Autodesk Inventor part; units mm, degrees
ref_plane "YZ Plane" through (0, 0, 0) normal (1, 0, 0) x (0, 1, 0)
ref_plane "XZ Plane" through (0, 0, 0) normal (0, 1, 0) x (-1, 0, 0)
ref_plane "XY Plane" through (0, 0, 0) normal (0, 0, 1) x (1, 0, 0)
sketch "Sketch4" plane through (0, 0, 0) normal (0, 1, 0) x (-1, 0, 0)
  line L0 (0, -20.574) -> (0, -15.748)
  line L1 (0, -15.748) -> (-3.302, -15.748)
  line L2 (-3.302, -15.748) -> (-3.302, -16.764)
  line L3 (-3.302, -16.764) -> (-10.2362, -16.764)
  line L4 (-10.2362, -16.764) -> (-10.2362, -20.574)
  line L5 (-10.2362, -20.574) -> (0, -20.574)
  line L6 (0, 0) -> (0, -4.826)
  line L7 (0, -4.826) -> (-3.302, -4.826)
  line L8 (-3.302, -4.826) -> (-3.302, -3.81)
  line L9 (-3.302, -3.81) -> (-10.2362, -3.81)
  line L10 (-10.2362, -3.81) -> (-10.2362, 0)
  line L11 (-10.2362, 0) -> (0, 0)
  dimension "d22" = 3.302
  dimension "d23" = 1.016
  dimension "d24" = 1.016
  dimension "d25" = 6.9342
  dimension "d26" = 3.81
  dimension "d27" = 20.574
  dimension "d28" = 3.81
extrude "Extrusion4" add sketch "Sketch4" along normal blind 10.8712
sketch "Sketch5" plane through (0, 0, 0) normal (0, -1, 0) x (1, 0, 0)
  line L0 (0, -15.748) -> (3.302, -15.748)
  line L1 (3.302, -15.748) -> (3.302, -4.826)
  line L2 (3.302, -4.826) -> (0, -4.826)
  line L3 (0, -4.826) -> (0, -15.748)
  line L4 (3.302, -4.826) -> (0, -4.826)
  line L5 (0, -15.748) -> (3.302, -15.748)
  line L6 (0, -20.574) -> (0, -15.748)
  line L7 (3.302, -15.748) -> (3.302, -16.764)
  point P0 (0, 0)
extrude "Extrusion5" add sketch "Sketch5" against normal blind 3.7592
pattern_linear "Rectangular Pattern2" count 8 spacing 10.2362 along (1, 0, 0) of "Extrusion4", "Extrusion5"
sketch "Sketch6" plane through (81.8896, 0, -16.764) normal (1, 0, 0) x (0, 0, -1)
  line L0 (3.81, 0) -> (-16.764, 0)
  line L1 (3.81, 10.8712) -> (-1.016, 10.8712)
  line L2 (3.81, 0) -> (3.81, 10.8712)
  line L3 (3.81, 10.8712) -> (-1.016, 10.8712)
  line L4 (-11.938, 3.7592) -> (-1.016, 3.7592)
  line L5 (-1.016, 10.8712) -> (-1.016, 3.7592)
  line L6 (-1.016, 3.7592) -> (-11.938, 3.7592)
  line L7 (-11.938, 3.7592) -> (-11.938, 10.8712)
  line L8 (-11.938, 3.7592) -> (-11.938, 10.8712)
  line L9 (-16.764, 0) -> (-16.764, 10.8712)
  line L10 (-11.938, 10.8712) -> (-16.764, 10.8712)
  line L11 (-16.764, 10.8712) -> (-16.764, 0)
  line L12 (3.81, 0) -> (-16.764, 0)
extrude "Extrusion6" add sketch "Sketch6" along normal blind 3.302
properties part number "LatchHolder"
Read the model definition and answer for the solid it produces. Units are mm, in the model's axes. A direction names the side the tool comes from. Give positions to 0.01 mm unless a question says otherwise; leave off trailing zeros. Loops run counter-clockwise (first coordinate to the right, second up) from the corner with the lowest first, then second, coordinate; pieces in that order, holes last.
Item 1: The part is cut by section B-B (x = 68). Write down the section's boundary in (y, z), and give its area (3 significant figures).
Item 2: Each of these flat-tipped pins is pushed along its axis until it touches: pin 1 Ø2.5 at (x, z) = (11.5, -10.5) entering from +Y; pin 2 Ø1.7 at (x, y) = (52.5, 7) entering from +Z; pin 3 Ø3.5 at (y, z) = (6, -11) entering from -X. Where does it stop, or does it pass through?
Item 3: For faces 1 (the flat face through (58, 5, -3.81)), 2 (the flat face through (84, 3.759, -10)), determine the directions among +Z, -Z, +X, -X, +Y, -Y from which every point of the face is accessible in a straight line to the end or side of a thin tool.
Item 4: Find the intervals of material crossed by line 1 along Z through (x, y) = (12, 8.75); line 2 along Z through (x, y) = (15, 7); line 3 along Y through (x, z) = (10.5, -6.5), in increasing order.
Item 5: The mould has two halves that part along Z. Classify faces 3 (the flat face through (37, 5, -16.764)), 4 (the flat face through (42, 10.871, -2)): released by +Z, released by -Z, zero draft, split by the parting line, or undercut.
Item 6: The part is cut by section C-C (z = -6.5). Give the number of separate pieces and of enclosed holes in the cut face, and give its area (3 significant figures).
Item 7: The part is cut by section A-A (x = 52). Write down the section's boundary in (y, z), and give its area (3 significant figures).
Taken from the geometry:
1. outline: (0, -20.57) - (10.87, -20.57) - (10.87, -16.76) - (0, -16.76) - close; (0, -3.81) - (10.87, -3.81) - (10.87, 0) - (0, 0) - close
1. area: 82.8 mm2
2. pin 1: stops at y = 3.76
2. pin 2: stops at z = 0
2. pin 3: passes through
3. face 1: +Y, -Y
3. face 2: +X, -X, +Y
4. line 1: z = -20.57 to -15.75, -4.83 to 0
4. line 2: z = -20.57 to -16.76, -3.81 to 0
4. line 3: y = 0 to 3.76
5. face 3: undercut
5. face 4: zero draft
6. separate pieces: 9
6. enclosed holes: 0
6. area: 112 mm2
7. outline: (0, -20.57) - (10.87, -20.57) - (10.87, -15.75) - (3.76, -15.75) - (3.76, -4.83) - (10.87, -4.83) - (10.87, 0) - (0, 0) - close
7. area: 146 mm2
